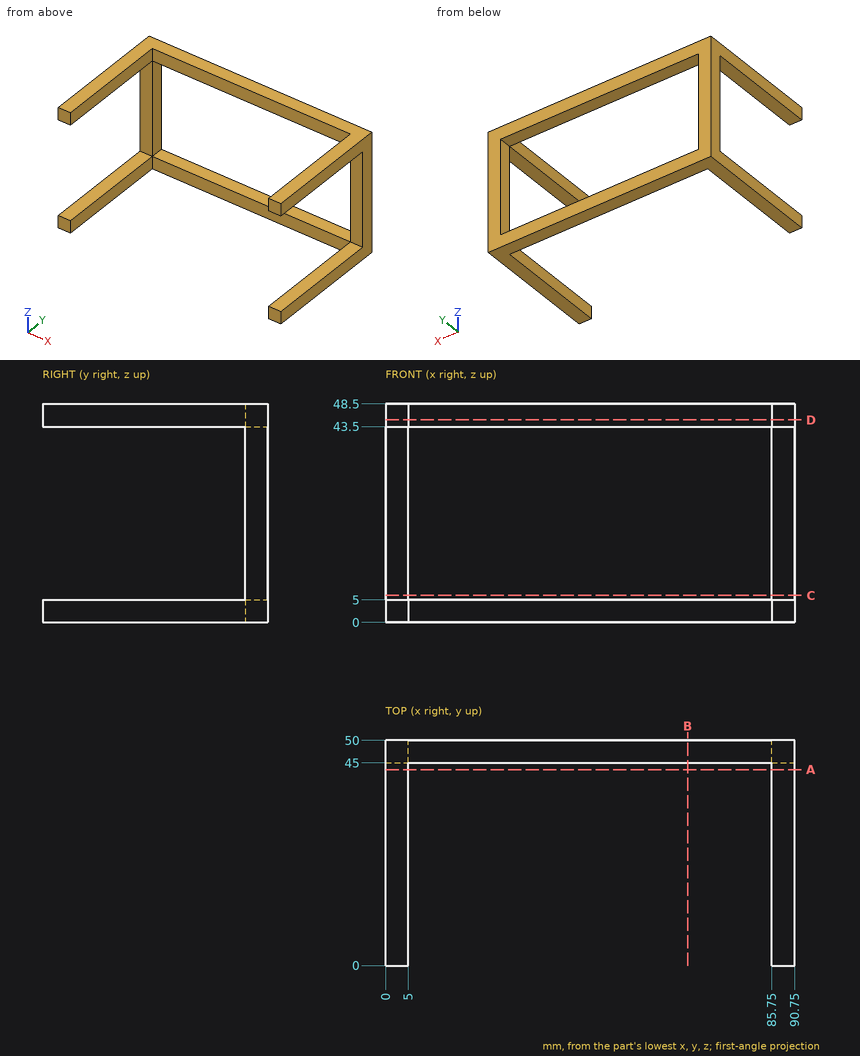
Check sheet for the drawn part. Datum: minimum x, y, z corner. Units: mm. Round coordinates to 2 decimals unless told otherwise and drop trailing zeros. Order: outer loops, then holes, each group sorted by start corner. A loop starts at its lowest first (then second) coordinate and runs counter-clockwise, first axis right, second up.
(1) Cross-section at B-B, the plane x = 67. Enter the section's corners in (y, z), and give its area (3 significant figures).
(2) Cross-section at A-A, the plane y = 43.5. Enter the section's corners in (x, z).
(3) Cross-section at D-D, the plane z = 45. Enter the section's corners in (x, y).
(4) Cross-section at C-C, the plane z = 6. Enter the section's corners in (x, y), and give its area (3 significant figures).
(5) Scan lines: probe 1 along X at (y, z) = (47, 32); probe 2 along Y at (x, z) = (77, 44). Record each from-to range of solid material in increasing order.
(6) Go/stop test with a flat-tipped pin: P1, Ø5.5, axis at x = 26, z = 3, coming from the -Y side. Record where the tip stops, or that it passes through.
Check sheet entries:
1. outline: (45, 0) - (50, 0) - (50, 5) - (45, 5) - close; (45, 43.5) - (50, 43.5) - (50, 48.5) - (45, 48.5) - close
1. area: 50.0 mm2
2. outline: (0, 0) - (5, 0) - (5, 5) - (0, 5) - close; (0, 43.5) - (5, 43.5) - (5, 48.5) - (0, 48.5) - close; (85.75, 0) - (90.75, 0) - (90.75, 5) - (85.75, 5) - close; (85.75, 43.5) - (90.75, 43.5) - (90.75, 48.5) - (85.75, 48.5) - close
3. outline: (0, 0) - (5, 0) - (5, 45) - (85.75, 45) - (85.75, 0) - (90.75, 0) - (90.75, 50) - (0, 50) - close
4. outline: (0, 45) - (5, 45) - (5, 50) - (0, 50) - close; (85.75, 45) - (90.75, 45) - (90.75, 50) - (85.75, 50) - close
4. area: 50.0 mm2
5. probe 1: x = 0 to 5, 85.75 to 90.75
5. probe 2: y = 45 to 50
6. P1: stops at y = 45
